```python
from build123d import *

# Parameters (mm, degrees)
BOSS_EXTRUDE1_DEPTH = 65


with BuildPart() as part:
    # Sketch1 → Boss-Extrude1 (new body, symmetric)
    with BuildSketch(Plane(origin=(0, 0, 0), x_dir=(0, 0, -1), z_dir=(1, 0, 0))):
        Polygon((1.555, 12.497186583), (3, 15), (0, 15), (-3, 15), (-1.555, 12.497186583), (-7.945, 12.497186583), (-6.5, 15), (-10, 15), (-10, -15), (10, -15), (10, 15), (6.5, 15), (7.945, 12.497186583), align=None)
    extrude(amount=BOSS_EXTRUDE1_DEPTH, both=True)


solid = part.part
```
Geometry check sheet. Reference: the model listing, model coordinates, mm. A direction names the side the tool comes from. Round coordinates to 2 decimals unless told otherwise and drop trailing zeros. Loops run counter-clockwise (first coordinate to the right, second up) from the corner with the lowest first, then second, coordinate; pieces in that order, holes last. Notation, with made-up numbers: M 60,66 L 85,66 A28 cw 85,101 Z; hole C -11.5,71.25 d2. An arc over 180 degrees is marked long. Return JSON: item names as keys, results as strings. Group by question number.
(1) Go/stop test with flat-tipped pins: pin 1 (1.9 mm diameter, centred on x = -8, z = -5.5, fed in from +Y); pin 2 (3 mm diameter, centred on x = -27.5, z = 4, fed in from +Y). Record where each tip stops, or that it passes through.
(2) Section check A-A, the plane x = 44. Enter the section's corners in (y, z) (3 decimals).
(3) Scan lines: line 1 along Y through (x, z) = (28, 5); line 2 along Y through (x, z) = (-56, -7.25); line 3 along Y through (x, z) = (-57.5, -7.5). Record each from-to range of solid material in increasing order. Write a range as [from, to].
(4) Mould release check, pull along Z, two halves, no side actions. Record for faces 1 (the face through (0.91, 13.77, 2.29)), 2 (the face through (1, 0, 10)), 3 (the face through (1, 0, -10)): pulls with the +Z half, pulls with the -Z half, needs draft (parallel to the pull), parting line crosses it, or undercut.
(5) Set-up check for faces 4 (the face through (1, 15, 8)), 5 (the face through (1, 12.497, -5)): record each of +Z, -Z, +X, -X, +Y, -Y from which the full face is reachable in a straight line by a thin tool's end or side.
Data:
{
 "1": {"pin 1": "y = 12.5", "pin 2": "y = 15"},
 "2": {"outline": "M -15,-10 L 15,-10 L 15,-6.5 L 12.497,-7.945 L 12.497,-1.555 L 15,-3 L 15,3 L 12.497,1.555 L 12.497,7.945 L 15,6.5 L 15,10 L -15,10 Z"},
 "3": {"line 1": "[-15, 12.5]", "line 2": "[-15, 12.5], [13.7, 15]", "line 3": "[-15, 12.5], [13.27, 15]"},
 "4": {"face 1": "undercut", "face 2": "pulls with the +Z half", "face 3": "pulls with the -Z half"},
 "5": {"face 4": "+Z, -Z, +X, -X, +Y", "face 5": "+X, -X"}
}
